Read the model definition and answer for the solid it produces. Units are mm, in the model's axes. Face numbers are marked on the shaded views. A direction names the side the tool comes from. Give positions to 0.01 mm unless a question says otherwise; leave off trailing zeros. Write each loop counter-clockwise with the first axis right and the second up, starting at its lowest first coordinate (ties: lowest second). Pieces come first, ordered by that corner, then holes. Notation, with made-up numbers: (7.25, 81.5) - (55.25, 81.5) arc R24 ccw to (55.25, 113.5) - close; hole circle Ø3 at (1, -5). An arc over 180 degrees is marked (long way). Use CSV: the item, a comma, the result in double quotes. Start each with the question number.
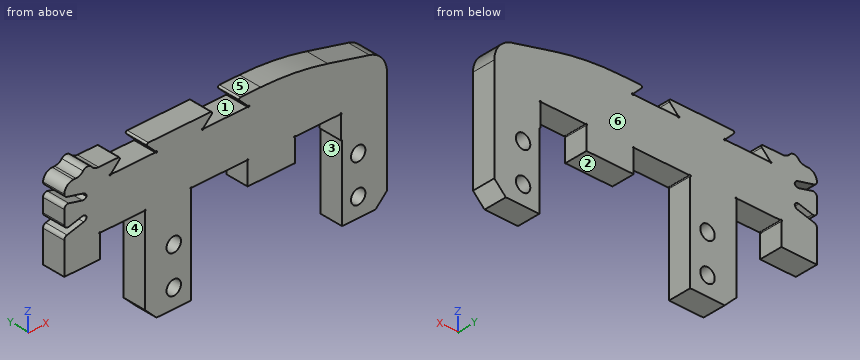
from build123d import *

# Parameters (mm, degrees)
BOSS_EXTRUDE1_DEPTH = 15.875
SKETCH3_W           = 12.7
SKETCH3_H           = 6.35
BOSS_EXTRUDE2_DEPTH = 26.9875
SKETCH5_R           = 1.5
BOSS_EXTRUDE4_DEPTH = 6.35
FILLET1_R           = 2.54
CUT_EXTRUDE1_DEPTH  = 62.570271083
FILLET3_R           = 1
CUT_EXTRUDE2_DEPTH  = 6.35
FILLET4_R           = 6.35
FILLET5_R           = 76.2
SKETCH8_W           = 9.825
SKETCH8_H           = 6.35
BOSS_EXTRUDE5_DEPTH = 6.35
SKETCH9_W           = 0.299999908
SKETCH9_H           = 20.6375
CUT_EXTRUDE3_DEPTH  = 62.570271083
FILLET6_R           = 2.54
FILLET7_R           = 2.54
SKETCH10_R          = 1.984375
CUT_EXTRUDE4_DEPTH  = 62.570271083
CHAMFER1_SIZE       = 3.175
SKETCH11_W          = 13
SKETCH11_H          = 6.35
BOSS_EXTRUDE6_DEPTH = 6.35
SKETCH12_R          = 0.1984375
CUT_EXTRUDE5_DEPTH  = 62.570271083
CUT_EXTRUDE6_DEPTH  = 6.35
FILLET8_R           = 0.396875
SKETCH14_R          = 0.1984375
CUT_EXTRUDE7_DEPTH  = 62.570271083
FILLET9_R           = 0.396875


with BuildPart() as part:
    # Sketch2 → Boss-Extrude1 (new body)
    with BuildSketch(Plane.XY):
        Polygon((51.8, -23.01875), (-33.925, -23.01875), (-33.925, -29.36875), (48.625, -29.36875), (54.975, -29.36875), (54.975, -23.01875), align=None)
    extrude(amount=BOSS_EXTRUDE1_DEPTH)

    # Sketch3 → Boss-Extrude2 (add)
    with BuildSketch(Plane(origin=(0, 0, 0), x_dir=(-1, 0, 0), z_dir=(0, 0, -1))):
        with Locations((5.35, -26.19375)):
            Rectangle(SKETCH3_W, SKETCH3_H)
        with Locations((-48.625, -26.19375)):
            Rectangle(SKETCH3_W, SKETCH3_H)
    extrude(amount=BOSS_EXTRUDE2_DEPTH)

    # Sketch5 → Boss-Extrude4 (add)
    with BuildSketch(Plane(origin=(0, -23.01875, 0), x_dir=(1, 0, 0), z_dir=(0, 1, 0))):
        with Locations((-27.575, -15.875)):
            Circle(SKETCH5_R)
    extrude(amount=-BOSS_EXTRUDE4_DEPTH)

    # Fillet1
    fillet1_edges = [part.edges().sort_by_distance(p)[0] for p in [
        (-26.075, -26.19375, 15.875),
    ]]
    fillet(fillet1_edges, radius=FILLET1_R)

    # Sketch6 → Cut-Extrude1 (cut, through all)
    with BuildSketch(Plane(origin=(0, -23.01875, 0), x_dir=(1, 0, 0), z_dir=(0, 1, 0))):
        Polygon((-33.925, -3.175), (-27.575, -4.7625), (-27.960025305, -6.302601219), (-34.310025305, -4.715101219), align=None)
        Polygon((-33.925, -12.7), (-27.575, -11.1125), (-27.960025305, -9.572398781), (-34.310025305, -11.159898781), align=None)
    extrude(amount=-CUT_EXTRUDE1_DEPTH, mode=Mode.SUBTRACT)

    # Fillet3
    # the kernel refuses this fillet: 1 mm, written as the material it adds along each edge
    with BuildSketch(Plane(origin=(-27.575, -23.01875, 11.1125), x_dir=(-0.24253562503632964, 0, -0.9701425001453328), z_dir=(0, -1, 0)), Plane(origin=(-27.960025305, -23.01875, 9.572398781), x_dir=(-0.970142500145332, 0, 0.242535625036333), z_dir=(0, -1, 0)), Plane(origin=(-27.960025305, -23.01875, 6.302601219), x_dir=(0.24253562503633191, 0, -0.9701425001453321), z_dir=(0, -1, 0)), Plane(origin=(-27.575, -23.01875, 4.7625), x_dir=(-0.9701425001453318, 0, -0.24253562503633383), z_dir=(0, -1, 0))) as fillet3_piece_1:
        with BuildLine():
            CenterArc((FILLET3_R, -FILLET3_R), FILLET3_R, 90, 90)
            Line((0, -FILLET3_R), (0, 0))
            Line((0, 0), (FILLET3_R, 0))
        make_face()
    extrude(amount=6.35)
    # the kernel refuses this fillet: 1 mm, written as the material it takes off along each edge
    with BuildSketch(Plane(origin=(-33.925, -21.066808984, 3.175), x_dir=(0, 0, -1), z_dir=(0, -1, 0)), Plane(origin=(-33.925, -21.066808984, 12.7), x_dir=(0.9701425001453319, 0, -0.24253562503633297), z_dir=(0, -1, 0))) as fillet3_2_piece_1:
        with BuildLine():
            CenterArc((FILLET3_R * 0.780776406404, FILLET3_R), FILLET3_R, 194.036243468, 75.963756532)
            Line((-FILLET3_R * 0.189366093741, FILLET3_R * 0.757464374964), (0, 0))
            Line((0, 0), (FILLET3_R * 0.780776406404, 0))
        make_face()
    extrude(amount=10.253882032, mode=Mode.SUBTRACT)
    with BuildSketch(Plane(origin=(-33.925, -32.570691016, 4.811357545), x_dir=(0.9701425001453321, 0, 0.24253562503633233), z_dir=(0, 1, 0)), Plane(origin=(-33.925, -32.570691016, 11.063642455), x_dir=(0, 0, -1), z_dir=(0, 1, 0))) as fillet3_2_piece_2:
        with BuildLine():
            CenterArc((FILLET3_R * 1.2807764064, -FILLET3_R), FILLET3_R, 90, 104.036243468)
            Line((FILLET3_R * 0.310633906259, -FILLET3_R * 1.24253562504), (0, 0))
            Line((0, 0), (FILLET3_R * 1.2807764064, 0))
        make_face()
    extrude(amount=12.753882032, mode=Mode.SUBTRACT)

    # Sketch7 → Cut-Extrude2 (cut)
    with BuildSketch(Plane(origin=(0, -29.36875, 0), x_dir=(-1, 0, 0), z_dir=(0, -1, 0))):
        Polygon((-54.975, -15.875), (-54.975, -9.525), (-29.575, -15.875), align=None)
    extrude(amount=-CUT_EXTRUDE2_DEPTH, mode=Mode.SUBTRACT)

    # Fillet4
    fillet4_edges = [part.edges().sort_by_distance(p)[0] for p in [
        (54.975, -26.19375, 9.525),
    ]]
    fillet(fillet4_edges, radius=FILLET4_R)

    # Fillet5
    fillet5_edges = [part.edges().sort_by_distance(p)[0] for p in [
        (29.575, -26.19375, 15.875),
    ]]
    fillet(fillet5_edges, radius=FILLET5_R)

    # Sketch8 → Boss-Extrude5 (add)
    with BuildSketch(Plane(origin=(0, 0, 0), x_dir=(-1, 0, 0), z_dir=(0, 0, -1))):
        with Locations((29.0125, -26.19375)):
            Rectangle(SKETCH8_W, SKETCH8_H)
    extrude(amount=BOSS_EXTRUDE5_DEPTH)

    # Sketch9 → Cut-Extrude3 (cut, through all)
    with BuildSketch(Plane(origin=(0, -23.01875, 0), x_dir=(1, 0, 0), z_dir=(0, 1, 0))):
        with Locations((42.424999954, 16.66875)):
            Rectangle(SKETCH9_W, SKETCH9_H)
    extrude(amount=-CUT_EXTRUDE3_DEPTH, mode=Mode.SUBTRACT)

    # Fillet6
    fillet6_edges = [part.edges().sort_by_distance(p)[0] for p in [
        (-29.075, -26.19375, 15.875),
    ]]
    fillet(fillet6_edges, radius=FILLET6_R)

    # Fillet7
    # the kernel refuses this fillet: 2.54 mm, written as the material it takes off along each edge
    with BuildSketch(Plane(origin=(-33.925, -16.679216678, 15.875), x_dir=(1, 0, 0), z_dir=(0, -1, 0))) as fillet7_piece_1:
        with BuildLine():
            CenterArc((2.535813329, -2.54), FILLET7_R, 90, 86.709856328)
            Line((0, -2.394223594), (-0.050716267, -2.391308065))
            ThreePointArc((-0.050716267, -2.391308065), (-0.0508, -1.197111797), (-0.0508, 0))
            Line((-0.0508, 0), (0, 0.0508))
            Line((0, 0.0508), (2.535813329, 0.0508))
            Line((2.535813329, 0.0508), (2.535813329, 0))
        make_face()
    extrude(amount=19.029066645, mode=Mode.SUBTRACT)

    # Sketch10 → Cut-Extrude4 (cut, through all)
    with BuildSketch(Plane(origin=(0, -29.36875, 0), x_dir=(-1, 0, 0), z_dir=(0, -1, 0))):
        with Locations(Location((-47.0375, 21.828125, 0), (0, 0, 180))):
            Circle(SKETCH10_R)
        with Locations(Location((-47.0375, 11.509375, 0), (0, 0, 180))):
            Circle(SKETCH10_R)
        with Locations(Location((3.7625, 11.509375, 0), (0, 0, 180))):
            Circle(SKETCH10_R)
        with Locations(Location((3.7625, 21.828125, 0), (0, 0, 180))):
            Circle(SKETCH10_R)
    extrude(amount=-CUT_EXTRUDE4_DEPTH, mode=Mode.SUBTRACT)

    # Chamfer1
    chamfer1_edges = [part.edges().sort_by_distance(p)[0] for p in [
        (54.975, -26.19375, -26.9875),
        (-11.7, -26.19375, -26.9875),
    ]]
    chamfer(chamfer1_edges, length=CHAMFER1_SIZE)

    # Sketch11 → Boss-Extrude6 (add)
    with BuildSketch(Plane(origin=(0, 0, 0), x_dir=(-1, 0, 0), z_dir=(0, 0, -1))):
        with Locations((-23.075, -26.19375)):
            Rectangle(SKETCH11_W, SKETCH11_H)
    extrude(amount=BOSS_EXTRUDE6_DEPTH)

    # Sketch12 → Cut-Extrude5 (cut, through all)
    with BuildSketch(Plane(origin=(0, -23.01875, 0), x_dir=(1, 0, 0), z_dir=(0, 1, 0))):
        with Locations((-24.1, 0)):
            Circle(SKETCH12_R)
        with Locations((-11.7, 0)):
            Circle(SKETCH12_R)
        with Locations((1, 0)):
            Circle(SKETCH12_R)
        with Locations((16.575, 0)):
            Circle(SKETCH12_R)
        with Locations((29.575, 0)):
            Circle(SKETCH12_R)
        with Locations((42.275, 0)):
            Circle(SKETCH12_R)
    extrude(amount=-CUT_EXTRUDE5_DEPTH, mode=Mode.SUBTRACT)

    # Sketch13 → Cut-Extrude6 (cut)
    with BuildSketch(Plane(origin=(0, -23.01875, 0), x_dir=(1, 0, 0), z_dir=(0, 1, 0))):
        Polygon((-21.225, -12.7), (-8.525, -12.7), (-11.7, -15.875), (-18.05, -15.875), align=None)
        Polygon((16.875, -12.7), (13.7, -15.875), (7.35, -15.875), (4.175, -12.7), align=None)
    extrude(amount=-CUT_EXTRUDE6_DEPTH, mode=Mode.SUBTRACT)

    # Fillet8
    fillet8_edges = [part.edges().sort_by_distance(p)[0] for p in [
        (-18.05, -26.19375, 15.875),
        (-11.7, -26.19375, 15.875),
        (7.35, -26.19375, 15.875),
        (13.7, -26.19375, 15.875),
    ]]
    fillet(fillet8_edges, radius=FILLET8_R)

    # Sketch14 → Cut-Extrude7 (cut, through all)
    with BuildSketch(Plane(origin=(0, -23.01875, 0), x_dir=(1, 0, 0), z_dir=(0, 1, 0))):
        with Locations((-21.225, -12.7)):
            Circle(SKETCH14_R)
        with Locations((-8.525, -12.7)):
            Circle(SKETCH14_R)
        with Locations((4.175, -12.7)):
            Circle(SKETCH14_R)
        with Locations((16.875, -12.7)):
            Circle(SKETCH14_R)
    extrude(amount=-CUT_EXTRUDE7_DEPTH, mode=Mode.SUBTRACT)

    # Fillet9
    fillet9_edges = [part.edges().sort_by_distance(p)[0] for p in [
        (-21.0265625, -26.19375, 12.7),
        (-21.084683498, -26.19375, 12.840316502),
        (-8.665316502, -26.19375, 12.840316502),
        (-8.7234375, -26.19375, 12.7),
        (4.3734375, -26.19375, 12.7),
        (4.315316502, -26.19375, 12.840316502),
        (16.734683498, -26.19375, 12.840316502),
        (16.6765625, -26.19375, 12.7),
    ]]
    fillet(fillet9_edges, radius=FILLET9_R)


solid = part.part
(1) The part is cut by section D-D on x = 24.5. Write down the section's boundary in (y, z), plus the area to 3 significant figures.
(2) The part is cut by section C-C on y = -24. Give the number of separate pieces and of enclosed holes in the cut face, plus the area to 3 significant figures.
(3) Given P1, Ø3, axis at x = 10, y = -26, coming from the +Z side; P2, Ø1.6, axis at x = -21, y = -27.5, coming from the +Z side (3 decimals), each flat-ended and moving along its own axis, determine where each tip first touches the part or whether it passes through.
(4) The part is cut by section A-A on z = -3. Write down the section's boundary in (x, y) (3 decimals), plus the area to 3 significant figures.
(5) For a pull along Z with two mould halves and no side action, classify the marked faces 1, 2 and 3 as pulls with the +Z half, pulls with the -Z half, needs draft (parallel to the pull), parting line crosses it, or undercut.
(6) The part is cut by section B-B on x = -16. Write down the section's boundary in (y, z), plus the area to 3 significant figures.
(7) Consider probe 1 along Z at (x, y) = (-3.5, -27.75) (1 decimal); probe 2 along X at (y, z) = (-27.5, -7.5) (3 decimals); probe 3 along Z at (x, y) = (46, -25). Determine where each line is inside the solid, lowest interval first.
(8) Which of the six approach directions +Z, -Z, +X, -X, +Y, -Y give full straight-line access (tool end or side, diameter ignored) to the marked faces 4, 5 and 6?
Reported:
1,outline,"(-29.37, -6.35) - (-23.02, -6.35) - (-23.02, 15.75) - (-29.37, 15.75) - close"
1,area,"140 mm²"
2,separate pieces,"1"
2,enclosed holes,"4"
2,area,"2,010 mm²"
3,P1,"z = 12.7"
3,P2,"z = 15.875"
4,outline,"(-33.925, -29.369) - (-24.1, -29.369) - (-24.1, -23.019) - (-33.925, -23.019) - close; (-11.7, -29.369) - (1, -29.369) - (1, -23.019) - (-11.7, -23.019) - close; (16.575, -29.369) - (29.575, -29.369) - (29.575, -23.019) - (16.575, -23.019) - close; (42.275, -29.369) - (54.975, -29.369) - (54.975, -23.019) - (42.275, -23.019) - close"
4,area,"306 mm²"
5,face 1,"undercut"
5,face 2,"pulls with the -Z half"
5,face 3,"needs draft"
6,outline,"(-29.37, 0) - (-23.02, 0) - (-23.02, 12.7) - (-29.37, 12.7) - close"
6,area,"80.6 mm²"
7,probe 1,"-27 to -23.8, -19.9 to -13.5, -9.5 to 15.9"
7,probe 2,"-11.7 to 1, 42.575 to 54.975"
7,probe 3,"-26.99 to -23.52, -20.14 to -13.2, -9.82 to 11.77"
8,face 4,"-Z, +Y, -Y"
8,face 5,"+Z, +X, +Y, -Y"
8,face 6,"+Z, -Z, +X, -X, +Y"
